```python
from build123d import *

# Parameters (mm, degrees)
F0_R     = 11.15
F1_DEPTH = 7


with BuildPart() as f1:
    # F0 (on Top) → F1 (new body)
    with BuildSketch(Plane.XY):
        with BuildLine():
            ThreePointArc((-11.503365, 19.928572), (-6.67601, 14.970685), (0, 13.15))
            ThreePointArc((0, 13.15), (6.453833, 14.842664), (11.246195, 19.484899))
            ThreePointArc((11.246195, 19.484899), (12.665109, 22.761989), (13.15, 26.3))
            ThreePointArc((13.15, 26.3), (-3.290384, 39.031688), (-11.503365, 19.928572))
        make_face()
        with Locations((0, 26.3)):
            Circle(F0_R, mode=Mode.SUBTRACT)
        with Locations((0, 26.3)):
            Circle(F0_R)
        with BuildLine():
            Line((-2.10331, 31.292442), (0, 33.447244))
            Line((0, 33.447244), (2.10331, 31.292442))
            ThreePointArc((2.10331, 31.292442), (1.145089, 29.736107), (2.851212, 29.080737))
            ThreePointArc((2.851212, 29.080737), (2.971602, 24.207772), (7.832865, 24.566114))
            ThreePointArc((7.832865, 24.566114), (5.252195, 19.77236), (0, 18.339049))
            ThreePointArc((0, 18.339049), (-5.252195, 19.77236), (-7.832865, 24.566114))
            ThreePointArc((-7.832865, 24.566114), (-2.971602, 24.207772), (-2.851212, 29.080737))
            ThreePointArc((-2.851212, 29.080737), (-1.145089, 29.736107), (-2.10331, 31.292442))
        make_face(mode=Mode.SUBTRACT)
        with BuildLine():
            ThreePointArc((0, 13.15), (6.608989, 11.368543), (11.427312, 6.506846))
            Line((11.427312, 6.506846), (11.246195, 19.484899))
            ThreePointArc((11.246195, 19.484899), (6.453833, 14.842664), (0, 13.15))
        make_face()
        with BuildLine():
            ThreePointArc((-11.095406, 7.057937), (-6.328927, 11.526803), (0, 13.15))
            ThreePointArc((0, 13.15), (-6.67601, 14.970685), (-11.503365, 19.928572))
            Line((-11.503365, 19.928572), (-11.095406, 7.057937))
        make_face()
        with BuildLine():
            ThreePointArc((11.388234, -6.575), (12.701925, -3.40347), (13.15, 0))
            ThreePointArc((13.15, 0), (12.772083, 3.129918), (11.660055, 6.079935))
            ThreePointArc((11.660055, 6.079935), (11.545657, 6.294466), (11.427312, 6.506846))
            ThreePointArc((11.427312, 6.506846), (6.608989, 11.368543), (0, 13.15))
            ThreePointArc((0, 13.15), (-6.328927, 11.526803), (-11.095406, 7.057937))
            ThreePointArc((-11.095406, 7.057937), (-11.223996, 6.851599), (-11.34875, 6.64292))
            ThreePointArc((-11.34875, 6.64292), (-13.149941, 0.039281), (-11.388234, -6.575))
            ThreePointArc((-11.388234, -6.575), (-6.81804, -11.244413), (-0.564649, -13.137872))
            ThreePointArc((-0.564649, -13.137872), (-0.321661, -13.146065), (-0.078562, -13.149765))
            ThreePointArc((-0.078562, -13.149765), (6.540952, -11.407824), (11.388234, -6.575))
        make_face()
        Circle(F0_R, mode=Mode.SUBTRACT)
        with BuildLine():
            ThreePointArc((11.660055, 6.079935), (12.772083, 3.129918), (13.15, 0))
            ThreePointArc((13.15, 0), (12.701925, -3.40347), (11.388234, -6.575))
            ThreePointArc((11.388234, -6.575), (16.302998, -1.703748), (23.010332, -0.00208))
            Line((23.010332, -0.00208), (11.660055, 6.079935))
        make_face()
        with BuildLine():
            ThreePointArc((23.010332, -0.00208), (16.302998, -1.703748), (11.388234, -6.575))
            ThreePointArc((11.388234, -6.575), (9.627208, -13.010516), (11.25132, -19.48194))
            ThreePointArc((11.25132, -19.48194), (26.045016, -25.887311), (35.926468, -13.15))
            ThreePointArc((35.926468, -13.15), (32.157241, -3.9346), (23.010332, -0.00208))
        make_face()
        with Locations((22.776468, -13.15)):
            Circle(F0_R, mode=Mode.SUBTRACT)
        with BuildLine():
            ThreePointArc((11.25132, -19.48194), (9.627208, -13.010516), (11.388234, -6.575))
            ThreePointArc((11.388234, -6.575), (6.540952, -11.407824), (-0.078562, -13.149765))
            Line((-0.078562, -13.149765), (11.25132, -19.48194))
        make_face()
        with Locations((22.776468, -13.15)):
            Circle(F0_R)
        with BuildLine():
            ThreePointArc((26.048395, -17.467741), (25.17968, -15.85973), (23.759051, -17.00959))
            ThreePointArc((23.759051, -17.00959), (19.478744, -14.677369), (17.358446, -19.066517))
            ThreePointArc((17.358446, -19.066517), (14.497269, -14.434714), (15.882082, -9.169525))
            ThreePointArc((15.882082, -9.169525), (19.749464, -5.337646), (25.191311, -5.499597))
            ThreePointArc((25.191311, -5.499597), (22.450346, -9.530403), (26.610263, -12.071147))
            ThreePointArc((26.610263, -12.071147), (26.324769, -13.876377), (28.151705, -13.824701))
            Line((28.151705, -13.824701), (28.966163, -16.723622))
            Line((28.966163, -16.723622), (26.048395, -17.467741))
        make_face(mode=Mode.SUBTRACT)
        with BuildLine():
            ThreePointArc((-22.497515, -0.002959), (-16.081041, -1.832149), (-11.388234, -6.575))
            ThreePointArc((-11.388234, -6.575), (-13.149941, 0.039281), (-11.34875, 6.64292))
            Line((-11.34875, 6.64292), (-22.497515, -0.002959))
        make_face()
        with BuildLine():
            Line((-11.506967, -19.926492), (-0.564649, -13.137872))
            ThreePointArc((-0.564649, -13.137872), (-6.81804, -11.244413), (-11.388234, -6.575))
            ThreePointArc((-11.388234, -6.575), (-10.074543, -9.74653), (-9.626468, -13.15))
            ThreePointArc((-9.626468, -13.15), (-10.105311, -16.666288), (-11.506967, -19.926492))
        make_face()
        with BuildLine():
            ThreePointArc((-9.626468, -13.15), (-10.074543, -9.74653), (-11.388234, -6.575))
            ThreePointArc((-11.388234, -6.575), (-16.081041, -1.832149), (-22.497515, -0.002959))
            ThreePointArc((-22.497515, -0.002959), (-34.290742, -19.501693), (-11.506967, -19.926492))
            ThreePointArc((-11.506967, -19.926492), (-10.105311, -16.666288), (-9.626468, -13.15))
        make_face()
        with Locations((-22.776468, -13.15)):
            Circle(F0_R, mode=Mode.SUBTRACT)
        with Locations((-22.776468, -13.15)):
            Circle(F0_R)
        with BuildLine():
            ThreePointArc((-28.151705, -13.824701), (-26.324769, -13.876377), (-26.610263, -12.071147))
            ThreePointArc((-26.610263, -12.071147), (-22.450346, -9.530403), (-25.191311, -5.499597))
            ThreePointArc((-25.191311, -5.499597), (-19.749464, -5.337646), (-15.882082, -9.169525))
            ThreePointArc((-15.882082, -9.169525), (-14.497269, -14.434714), (-17.358446, -19.066517))
            ThreePointArc((-17.358446, -19.066517), (-19.478744, -14.677369), (-23.759051, -17.00959))
            ThreePointArc((-23.759051, -17.00959), (-25.17968, -15.85973), (-26.048395, -17.467741))
            Line((-26.048395, -17.467741), (-28.966163, -16.723622))
            Line((-28.966163, -16.723622), (-28.151705, -13.824701))
        make_face(mode=Mode.SUBTRACT)
    extrude(amount=F1_DEPTH)


solid = f1.part
```
Input: part model. Units: mm. Frame: model coordinates. A direction names the side the tool comes from. Give positions to 0.01 mm unless a question says otherwise; leave off trailing zeros. Order: outer loops, then holes, each group sorted by start corner. A loop starts at its lowest first (then second) coordinate and runs counter-clockwise, first axis right, second up. Notation, with made-up numbers: (-24.5, 70) - (-5.5, 70) arc R14 ccw to (-5.5, 93) - close; hole circle Ø11 at (-12, 88). An arc over 180 degrees is marked (long way). Put each result on its own line as item: value.
Item 1: Access query for faces 1 (the cylindrical face through (10.635, 3.349, 3.451)), 2 (the flat face through (5.507, -16.272, 3.451)). Directions: +Z, -Z, +X, -X, +Y, -Y. A direction counts if a zero-diameter tool reaches every point of the face in a straight line with its end or side. Return the directions, or none.
Found:
face 1: +Z, -Z
face 2: +Z, -Z, -Y
Item 2: Section query B-B, the plane y = -10. Return loops of the section in (x, z), then the cut area to 3 significant figures.
Found:
outline: (-35.54, 0) - (-22.59, 0) - (-22.59, 7) - (-35.54, 7) - close; (-15.33, 0) - (-4.93, 0) - (-4.93, 7) - (-15.33, 7) - close; (4.93, 0) - (15.33, 0) - (15.33, 7) - (4.93, 7) - close; (22.59, 0) - (35.54, 0) - (35.54, 7) - (22.59, 7) - close
area: 327 mm^2
Item 3: Section query C-C, the plane y = 3.5. Return loops of the section in (x, z), then the cut area to 3 significant figures.
Found:
outline: (-16.62, 0) - (-10.59, 0) - (-10.59, 7) - (-16.62, 7) - close; (10.59, 0) - (16.47, 0) - (16.47, 7) - (10.59, 7) - close
area: 83.5 mm^2
Item 4: Section query D-D, the plane x = -6. Return loops of the section in (y, z).
Found:
outline: (-16.51, 0) - (-9.4, 0) - (-9.4, 7) - (-16.51, 7) - close; (9.4, 0) - (20.46, 0) - (20.46, 7) - (9.4, 7) - close; (23.42, 0) - (38, 0) - (38, 7) - (23.42, 7) - close
Item 5: Draft query along X for faces 3 (the flat face through (-8, -8, 0)), 4 (the cylindrical face through (-34.472, -19.161, 3.451)). Return one class per face: +X half, -X half, draft (parallel to the pull), parting line (faces both ways), or undercut.
Found:
face 3: draft
face 4: undercut
Item 6: Section query A-A, the plane x = 9.5. Return loops of the section in (y, z).
Found:
outline: (-18.5, 0) - (-5.84, 0) - (-5.84, 7) - (-18.5, 7) - close; (5.84, 0) - (35.39, 0) - (35.39, 7) - (5.84, 7) - close
Item 7: Ray query, L1, parallel to X at y = -13.5, z = 6.25; L2, parallel to Y at x = -7, z = 2.5; L3, parallel to Y at x = -24.5, z = 5.25. Return the intervals inside material, ascending. Write a range as from..to.
Found:
L1: x = -35.92..-26.1, -14.42..-1.15, 0.55..14.42, 26.1..35.92
L2: y = -17.13..-8.68, 8.68..21.84, 23.84..37.43
L3: y = -26.19..-15.92, -11.95..-5.69, -5.22..-0.11
Item 8: Contact query for flat-ended pins moving along their axis: pin 1 (4 mm diameter, centred on x = -25.5, z = 3, fed in from -Y); pin 2 (1 mm diameter, centred on x = 17.5, z = 3.5, fed in from -Y); pin 3 (1 mm diameter, centred on x = -11.5, z = 6, fed in from +Y). Output: stop coordinate, or through.
Found:
pin 1: stops at y = -26.28
pin 2: stops at y = -25.4
pin 3: stops at y = 33.51
